```python
from build123d import *

# Parameters (mm, degrees)
SKETCH1_R           = 3.5
BOSS_EXTRUDE1_DEPTH = 5
SKETCH2_R           = 2
BOSS_EXTRUDE2_DEPTH = 5
CUT_EXTRUDE1_DEPTH  = 1.25


with BuildPart() as part:
    # Sketch1 → Boss-Extrude1 (new body)
    with BuildSketch(Plane(origin=(-2.712826585, 0, 0), x_dir=(0, 0, -1), z_dir=(1, 0, 0))):
        with BuildLine():
            ThreePointArc((-81.947812788, 41.849675859), (-81.477011433, 40.124136701), (-80.275497155, 38.799182837))
            ThreePointArc((-80.275497155, 38.799182837), (-80.771500839, 38.155576831), (-81.197397579, 37.463579494))
            ThreePointArc((-81.197397579, 37.463579494), (-82.862313797, 38.117179744), (-84.642669398, 37.94550204))
            ThreePointArc((-84.642669398, 37.94550204), (-84.747423061, 37.679683216), (-84.845284304, 37.411250441))
            ThreePointArc((-84.845284304, 37.411250441), (-83.626512376, 36.102153696), (-81.946887557, 35.48733684))
            ThreePointArc((-81.946887557, 35.48733684), (-82.086978383, 34.686947618), (-82.14250402, 33.876290323))
            ThreePointArc((-82.14250402, 33.876290323), (-83.920457299, 33.681299457), (-85.417101287, 32.701913897))
            ThreePointArc((-85.417101287, 32.701913897), (-85.386323881, 32.417861562), (-85.348228779, 32.134697757))
            ThreePointArc((-85.348228779, 32.134697757), (-83.660692239, 31.541941712), (-81.887738682, 31.778108996))
            ThreePointArc((-81.887738682, 31.778108996), (-81.63982353, 31.004296084), (-81.31225781, 30.260690647))
            ThreePointArc((-81.31225781, 30.260690647), (-82.795940481, 29.261778722), (-83.666009754, 27.699050735))
            ThreePointArc((-83.666009754, 27.699050735), (-83.506752013, 27.461837857), (-83.341427693, 27.228812437))
            ThreePointArc((-83.341427693, 27.228812437), (-81.571720826, 27.488190359), (-80.111600825, 28.521238704))
            ThreePointArc((-80.111600825, 28.521238704), (-79.532474069, 27.951273314), (-78.896858351, 27.44507078))
            ThreePointArc((-78.896858351, 27.44507078), (-79.746376594, 25.871076479), (-79.790548767, 24.083008214))
            ThreePointArc((-79.790548767, 24.083008214), (-79.53929472, 23.946977405), (-79.284614992, 23.817473685))
            ThreePointArc((-79.284614992, 23.817473685), (-77.838156313, 24.869565218), (-77.025365765, 26.462835698))
            ThreePointArc((-77.025365765, 26.462835698), (-76.247698364, 26.227290032), (-75.44964455, 26.074455301))
            ThreePointArc((-75.44964455, 26.074455301), (-75.470383973, 24.285961751), (-74.678539734, 22.682178099))
            ThreePointArc((-74.678539734, 22.682178099), (-74.392848655, 22.678492377), (-74.107157575, 22.682178099))
            ThreePointArc((-74.107157575, 22.682178099), (-73.315313337, 24.285961751), (-73.33605276, 26.074455301))
            ThreePointArc((-73.33605276, 26.074455301), (-72.537998945, 26.227290032), (-71.760331544, 26.462835698))
            ThreePointArc((-71.760331544, 26.462835698), (-70.947540996, 24.869565218), (-69.501082317, 23.817473685))
            ThreePointArc((-69.501082317, 23.817473685), (-69.246402589, 23.946977405), (-68.995148542, 24.083008214))
            ThreePointArc((-68.995148542, 24.083008214), (-69.039320715, 25.871076479), (-69.888838958, 27.44507078))
            ThreePointArc((-69.888838958, 27.44507078), (-69.25322324, 27.951273314), (-68.674096484, 28.521238704))
            ThreePointArc((-68.674096484, 28.521238704), (-67.213976483, 27.488190359), (-65.444269616, 27.228812437))
            ThreePointArc((-65.444269616, 27.228812437), (-65.278945296, 27.461837857), (-65.119687555, 27.699050735))
            ThreePointArc((-65.119687555, 27.699050735), (-65.989756828, 29.261778722), (-67.473439499, 30.260690647))
            ThreePointArc((-67.473439499, 30.260690647), (-67.145873779, 31.004296084), (-66.897958627, 31.778108996))
            ThreePointArc((-66.897958627, 31.778108996), (-65.12500507, 31.541941712), (-63.437468531, 32.134697757))
            ThreePointArc((-63.437468531, 32.134697757), (-63.399373428, 32.417861562), (-63.368596022, 32.701913897))
            ThreePointArc((-63.368596022, 32.701913897), (-64.86524001, 33.681299457), (-66.643193289, 33.876290323))
            ThreePointArc((-66.643193289, 33.876290323), (-66.698718926, 34.686947618), (-66.838809753, 35.48733684))
            ThreePointArc((-66.838809753, 35.48733684), (-65.159184933, 36.102153696), (-63.940413005, 37.411250441))
            ThreePointArc((-63.940413005, 37.411250441), (-64.038274248, 37.679683216), (-64.143027911, 37.94550204))
            ThreePointArc((-64.143027911, 37.94550204), (-65.923383512, 38.117179744), (-67.58829973, 37.463579494))
            ThreePointArc((-67.58829973, 37.463579494), (-68.01419647, 38.155576831), (-68.510200154, 38.799182837))
            ThreePointArc((-68.510200154, 38.799182837), (-67.308685876, 40.124136701), (-66.837884521, 41.849675859))
            ThreePointArc((-66.837884521, 41.849675859), (-67.049283279, 42.041882889), (-67.265570208, 42.228572314))
            ThreePointArc((-67.265570208, 42.228572314), (-68.92177941, 41.55321287), (-70.092246326, 40.200753443))
            ThreePointArc((-70.092246326, 40.200753443), (-70.790946358, 40.615562571), (-71.529234434, 40.954942982))
            ThreePointArc((-71.529234434, 40.954942982), (-71.081083139, 42.686502891), (-71.466107273, 44.433184235))
            ThreePointArc((-71.466107273, 44.433184235), (-71.742614638, 44.505133207), (-72.020886105, 44.569924936))
            ThreePointArc((-72.020886105, 44.569924936), (-73.173531339, 43.202245052), (-73.581409088, 41.460758605))
            ThreePointArc((-73.581409088, 41.460758605), (-74.392848655, 41.503351752), (-75.204288221, 41.460758605))
            ThreePointArc((-75.204288221, 41.460758605), (-75.61216597, 43.202245052), (-76.764811205, 44.569924936))
            ThreePointArc((-76.764811205, 44.569924936), (-77.043082671, 44.505133207), (-77.319590036, 44.433184235))
            ThreePointArc((-77.319590036, 44.433184235), (-77.70461417, 42.686502891), (-77.256462875, 40.954942982))
            ThreePointArc((-77.256462875, 40.954942982), (-77.994750951, 40.615562571), (-78.693450983, 40.200753443))
            ThreePointArc((-78.693450983, 40.200753443), (-79.863917899, 41.55321287), (-81.520127101, 42.228572314))
            ThreePointArc((-81.520127101, 42.228572314), (-81.73641403, 42.041882889), (-81.947812788, 41.849675859))
        make_face()
        with Locations((-74.392848655, 33.752711127)):
            Circle(SKETCH1_R, mode=Mode.SUBTRACT)
    extrude(amount=-BOSS_EXTRUDE1_DEPTH)

    # Sketch2 → Boss-Extrude2 (add)
    with BuildSketch(Plane(origin=(-2.712826585, 0, 0), x_dir=(0, 0, -1), z_dir=(1, 0, 0))):
        with BuildLine():
            Line((-36.340788792, 9.544432787), (-71.164417227, 35.104462035))
            ThreePointArc((-71.164417227, 35.104462035), (-71.527272682, 31.649420661), (-74.714649395, 30.267536198))
            Line((-74.714649395, 30.267536198), (-39.891020959, 4.70750695))
            ThreePointArc((-39.891020959, 4.70750695), (-35.697441957, 5.350853784), (-36.340788792, 9.544432787))
        make_face()
        with Locations((-38.115904876, 7.125969868)):
            Circle(SKETCH2_R, mode=Mode.SUBTRACT)
    extrude(amount=-BOSS_EXTRUDE2_DEPTH)

    # Sketch4 → Cut-Extrude1 (cut)
    with BuildSketch(Plane(origin=(-2.712826585, 0, 0), x_dir=(0, 0, -1), z_dir=(1, 0, 0))):
        with BuildLine():
            Line((-0.915831104, -5.866675378), (-4.542476407, -4.193411072))
            ThreePointArc((-4.542476407, -4.193411072), (-3.521318412, -6.746986699), (-0.915831104, -5.866675378))
        make_face()
        with BuildLine():
            ThreePointArc((-70.977992994, 34.520018639), (-71.581978602, 31.667283222), (-74.137028803, 30.262072761))
            Line((-74.137028803, 30.262072761), (-64.084174194, 23.709202076))
            Line((-64.084174194, 23.709202076), (-61.723827508, 26.931178659))
            Line((-61.723827508, 26.931178659), (-70.977992994, 34.520018639))
        make_face()
        with BuildLine():
            Line((-61.723827508, 26.931178659), (-64.084174194, 23.709202076))
            ThreePointArc((-64.084174194, 23.709202076), (-61.378637545, 24.202743939), (-61.723827508, 26.931178659))
        make_face()
    extrude(amount=-CUT_EXTRUDE1_DEPTH, mode=Mode.SUBTRACT)


solid = part.part
```
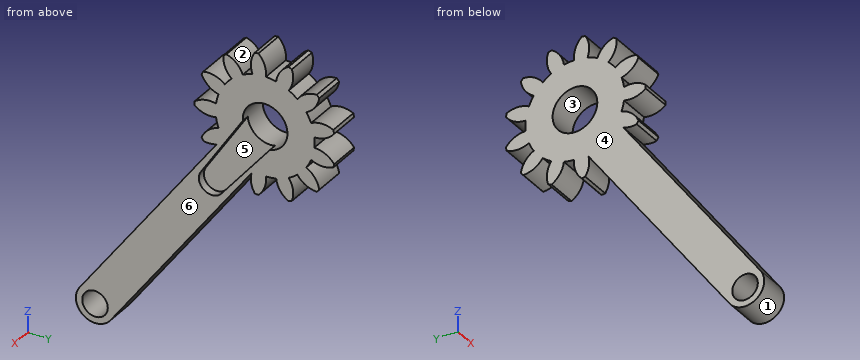
Design review of the part built by this model. Coordinates are the model's own, in mm. Face numbers are marked on the shaded views. A direction names the side the tool comes from. Coordinates: 2 decimals unless noted, no trailing zeros. Write each loop counter-clockwise with the first axis right and the second up, starting at its lowest first coordinate (ties: lowest second). Pieces come first, ordered by that corner, then holes. Notation, with made-up numbers: M 57.25,9.25 L 88.25,9.25 A35 ccw 88.25,45.25 Z; hole C -17,88 d1. An arc over 180 degrees is marked long. Answer as a JSON object with one key per item and string values.
Item 1: Add section C-C, the plane z = 47. Give the boundary of the cut face in (x, y).
Outcome:
{"outline": "M -7.71,9.93 L -2.71,9.93 L -2.71,17.37 L -7.71,17.37 Z"}
Item 2: Add section A-A, the plane x = -5.35. State how many separate pieces and enclosed holes the cut face has, and give its area (3 significant figures).
Outcome:
{"separate pieces": "1", "enclosed holes": "2", "area": "453 mm²"}
Item 3: Wall thickness on probe 1 along Y at (x, z) = (-7.25, 81.5); probe 2 along Z at (x, y) = (-4.05, 32.5); probe 3 along Z at (x, y) = (-4.75, 25): over which ranges is each line inside the solid? List them lowest first.
Outcome:
{"probe 1": "27.52 to 30.18, 30.66 to 37.65, 40.17 to 42.23", "probe 2": "63.39 to 71.12, 77.66 to 85.4", "probe 3": "57.4 to 67.54, 68.91 to 71.05, 73.22 to 75.56, 77.73 to 79.87"}
Item 4: Machinability: for the marked faces 5 and 6, which of the approach directions +Z, -Z, +X, -X, +Y, -Y give a long, thin tool a straight path to every point of the face, cutting with its end or side? Answer none if there is none.
Outcome:
{"face 5": "+X", "face 6": "+Z, -Z, +X, +Y, -Y"}
Item 5: Draft analysis for pull direction Y (two halves, no side actions). For the marked faces 1, 2, 3 and 4, state which applies: pulls with the +Y half, pulls with the -Y half, needs draft (parallel to the pull), parting line crosses it, or undercut.
Outcome:
{"face 1": "parting line crosses it", "face 2": "undercut", "face 3": "undercut", "face 4": "needs draft"}
Item 6: Add section B-B, the plane y = 14. Give the boundary of the cut face in (x, z).
Outcome:
{"outline": "M -7.71,42.41 L -2.71,42.41 L -2.71,52.55 L -7.71,52.55 Z"}
